CAD build for the part. Positions are in the model's coordinates, mm. Give positions to 0.01 mm unless a question says otherwise; leave off trailing zeros. Write each loop counter-clockwise with the first axis right and the second up, starting at its lowest first coordinate (ties: lowest second). Pieces come first, ordered by that corner, then holes. Notation, with made-up numbers: (54.25, -14) - (105.25, -14) arc R31 cw to (105.25, 13) - close; hole circle Ø5 at (-7, -29.5). An arc over 180 degrees is marked (long way). Answer as a JSON object with one key per item and string values.
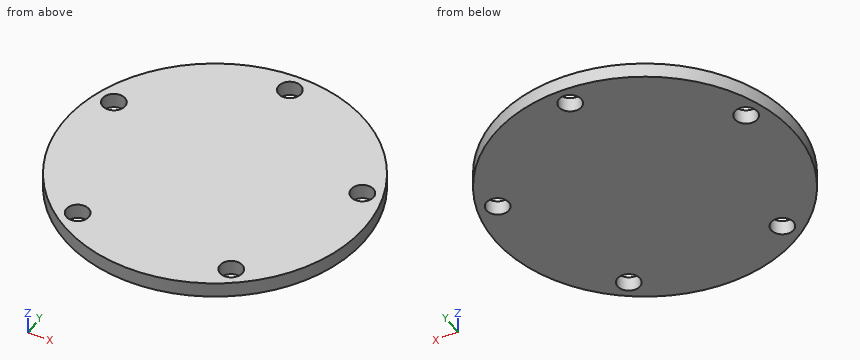
Autodesk Inventor part; units mm, degrees
ref_plane "YZ Plane" through (0, 0, 0) normal (1, 0, 0) x (0, 1, 0)
ref_plane "XZ Plane" through (0, 0, 0) normal (0, 1, 0) x (-1, 0, 0)
ref_plane "XY Plane" through (0, 0, 0) normal (0, 0, 1) x (1, 0, 0)
sketch "Sketch1" plane through (0, 0, 0) normal (0, 0, 1) x (1, 0, 0)
  circle A0 centre (0, 0) radius 20
  dimension "d0" = 40
extrude "Extrusion1" add sketch "Sketch1" along normal blind 2
sketch "Sketch2" plane through (0, 0, 2) normal (0, 0, 1) x (1, 0, 0)
  circle A0 centre (0, 0) radius 17.5 construction
  point P0 (0, 17.5)
  dimension "d3" = 35
hole "Hole1" at (0, 17.5, 2) direction (0, 0, -1) diameter 3 depth 2
pattern_circular "Circular Pattern1" count 5 over 360 about axis through (0, 0, 0) along (0, 0, 1) of "Hole1"
properties part number "35" material "Copper, Alloy"
(1) Flat gauge pins, fed straight in: P1, Ø1, axis at y = -6, z = 0.5, coming from the -X side; P2, Ø1, axis at y = 10, z = 0.5, coming from the +X side. Where does each tip first touch, or does it go through?
Answer key:
{"P1": "stops at x = -19.23", "P2": "stops at x = 17.6"}
(2) Saw through at D-D, the plane x = 7.5. Give the cut face in (y, z), and give its area (3 significant figures).
Answer key:
{"outline": "(-18.54, 0) - (18.54, 0) - (18.54, 2) - (-18.54, 2) - close", "area": "74.2 mm²"}
(3) Saw through at A-A, the plane x = 0. Give the cut face in (y, z), and give its area (3 significant figures).
Answer key:
{"outline": "(-20, 0) - (16, 0) - (16, 2) - (-20, 2) - close; (19, 0) - (20, 0) - (20, 2) - (19, 2) - close", "area": "74.0 mm²"}
(4) Saw through at B-B, the plane y = 17.5. Give the cut face in (x, z), and give its area (3 significant figures).
Answer key:
{"outline": "(-9.68, 0) - (-1.5, 0) - (-1.5, 2) - (-9.68, 2) - close; (1.5, 0) - (9.68, 0) - (9.68, 2) - (1.5, 2) - close", "area": "32.7 mm²"}
(5) Probe L1, parallel to Y at x = 0, z = 1.15; L2, parallel to X at y = -13, z = 0.3; L3, parallel to Y at x = -17, z = 0.7. List the from-to ranges inside material, lowest first. Write a range as [from, to].
Answer key:
{"L1": "y = [-20, 16], [19, 20]", "L2": "x = [-15.2, -11.24], [-9.33, 9.33], [11.24, 15.2]", "L3": "y = [-10.54, 3.95], [6.86, 10.54]"}
